The drawing under review shows one solid part. Ordinate dimensions are in mm from its lowest x, y, z. Coordinates: 2 decimals unless noted, no trailing zeros. Loops run counter-clockwise (first coordinate to the right, second up) from the corner with the lowest first, then second, coordinate; pieces in that order, holes last.
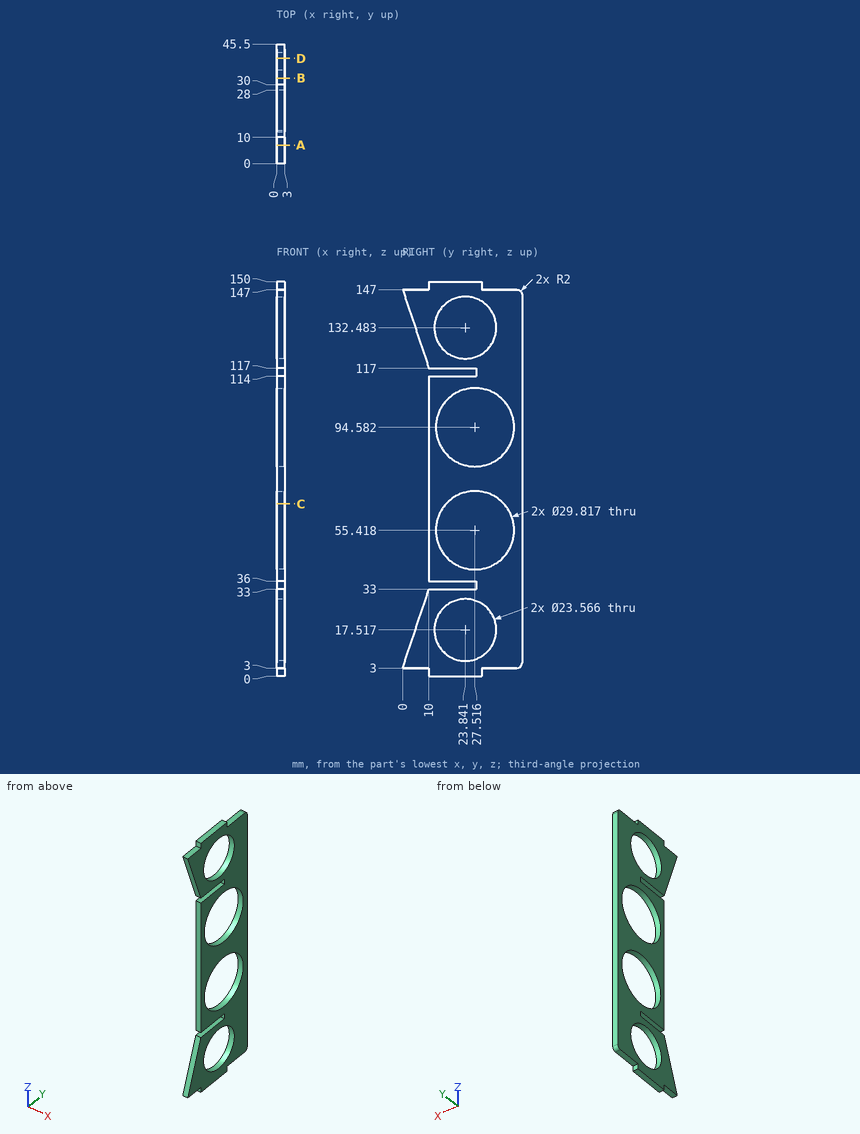
Q1. Take a section at D-D, the plane y = 40. Write out the cut boundary in (x, z).
Q2. Clearance check with flat-ended pins moving along their axes: pin 1 Ø1.5 at (x, y) = (1, 16.5) entering from -Z; pin 2 Ø0.9 at (x, y) = (1.5, 36) entering from -Z; pin 3 Ø1.5 at (x, y) = (1, 5) entering from +Z; pin 4 Ø1.5 at (x, z) = (1.5, 120.5) entering from -Y. State where each tip first meets the part, or that it passes through.
Q3. Take a section at C-C, the plane z = 65.5. Write out the cut boundary in (x, y).
Q4. For line 1 (Z direction, x = 1.6, y = 41) (1 decimal); line 2 (Z direction, x = 1.35, y = 29) (1 decimal); line 3 (Z direction, x = 2.1, y = 33) (1 decimal), list the stretches that pass through material, from the lowest coordinate up.
Q5. Take a section at A-A, the plane y = 7. Write out the cut boundary in (x, z), then the cut area to 3 significant figures.
Q6. Take a section at B-B, the plane y = 32.5. Write out the cut boundary in (x, z) (1 decimal).
Entries:
1. outline: (0, 3) - (3, 3) - (3, 47.27) - (0, 47.27) - close; (0, 63.57) - (3, 63.57) - (3, 86.43) - (0, 86.43) - close; (0, 102.73) - (3, 102.73) - (3, 147) - (0, 147) - close
2. pin 1: stops at z = 0
2. pin 2: stops at z = 3
2. pin 3: stops at z = 147
2. pin 4: stops at y = 8.58
3. outline: (0, 10) - (3, 10) - (3, 16.53) - (0, 16.53) - close; (0, 38.5) - (3, 38.5) - (3, 45.5) - (0, 45.5) - close
4. line 1: z = 3 to 49.1, 61.8 to 88.2, 100.9 to 147
4. line 2: z = 0 to 6.9, 28.1 to 40.6, 70.3 to 79.7, 109.4 to 121.9, 143.1 to 150
4. line 3: z = 3 to 10.1, 24.9 to 41.6, 69.3 to 80.7, 108.4 to 125.1, 139.9 to 147
5. outline: (0, 3) - (3, 3) - (3, 24) - (0, 24) - close; (0, 126) - (3, 126) - (3, 147) - (0, 147) - close
5. area: 126 mm2
6. outline: (0, 3) - (3, 3) - (3, 9.5) - (0, 9.5) - close; (0, 25.5) - (3, 25.5) - (3, 41.4) - (0, 41.4) - close; (0, 69.5) - (3, 69.5) - (3, 80.5) - (0, 80.5) - close; (0, 108.6) - (3, 108.6) - (3, 124.5) - (0, 124.5) - close; (0, 140.5) - (3, 140.5) - (3, 147) - (0, 147) - close
